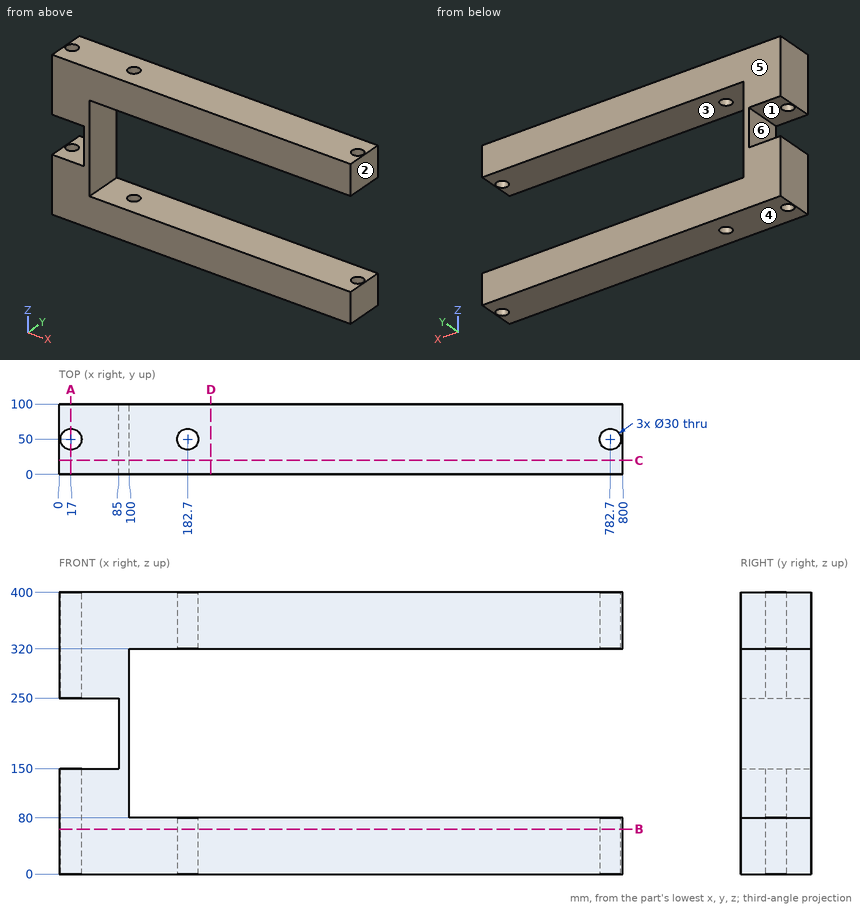
Here's the drawing with two shaded views (mm, measured from the low corner). I have some questions. A direction names the side the tool comes from. Give positions to 0.01 mm unless a question says otherwise; leave off trailing zeros. Loops run counter-clockwise (first coordinate to the right, second up) from the corner with the lowest first, then second, coordinate; pieces in that order, holes last. Notation, with made-up numbers: M 35.25,-36.75 L 75.25,-36.75 A12 cw 75.25,-29.75 Z; hole C 1,-11 d2. An arc over 180 degrees is marked long. Use one line per item in the form item = value. Start each with the question number.
Q1. Will these pins go through, and if not, where does the flat tip stop? pin 1 Ø5 at (y, z) = (69.5, 263.5) entering from -X; pin 2 Ø8 at (y, z) = (24.5, 212) entering from -X.
Q2. Thinking about a two-plate mould opening in Z: for the marked faces 4, 5 and 6, which applies, +Z half, -Z half, draft (parallel to the pull), parting line (faces both ways), or undercut?
Q3. I need wall thicknesses on line 1 along X through (y, z) = (50, 370); line 2 along Z through (x, y) = (466.5, 84); line 3 along Z through (x, y) = (33, 30). Which ranges of each line are inside material? Lowest first, please.
Q4. If we section it at D-D (x = 215.5): Write out the boundary of the cut face in (y, z).
Q5. If we section it at C-C (y = 20): Write out the boundary of the cut face in (x, z).
Q6. If we section it at A-A (x = 17): Write out the boundary of the cut face in (y, z), then the cut area to 3 significant figures.
Q7. If we section it at B-B (z = 64): Write out the boundary of the cut face in (x, y), then the cut area to 3 significant figures.
Q8. Which directions (+Z, -Z, +X, -X, +Y, -Y) give clear straight access to the entire face, cutting with the end or side of a thin tool? Please do the marked faces 1, 2 and 3.
Taken from the geometry:
q1.pin_1 = 0
q1.pin_2 = 85
q2.face_4 = -Z half
q2.face_5 = draft
q2.face_6 = undercut
q3.line_1 = 0 to 2, 32 to 167.7, 197.7 to 767.7, 797.7 to 800
q3.line_2 = 0 to 80, 320 to 400
q3.line_3 = 0 to 150, 250 to 400
q4.outline = M 0,0 L 100,0 L 100,80 L 0,80 Z; M 0,320 L 100,320 L 100,400 L 0,400 Z
q5.outline = M 0,0 L 800,0 L 800,80 L 100,80 L 100,320 L 800,320 L 800,400 L 0,400 L 0,250 L 85,250 L 85,150 L 0,150 Z
q6.outline = M 0,0 L 35,0 L 35,150 L 0,150 Z; M 0,250 L 35,250 L 35,400 L 0,400 Z; M 65,0 L 100,0 L 100,150 L 65,150 Z; M 65,250 L 100,250 L 100,400 L 65,400 Z
q6.area = 21,000 mm^2
q7.outline = M 0,0 L 800,0 L 800,100 L 0,100 Z; hole C 17,50 d30; hole C 182.7,50 d30; hole C 782.7,50 d30
q7.area = 77,900 mm^2
q8.face_1 = -X, +Y, -Y
q8.face_2 = +Z, -Z, +X, +Y, -Y
q8.face_3 = +X, +Y, -Y
